Work out the finished part from the listing and answer in its coordinate system (mm). A direction names the side the tool comes from. Round coordinates to 2 decimals unless told otherwise and drop trailing zeros. Write each loop counter-clockwise with the first axis right and the second up, starting at its lowest first coordinate (ties: lowest second). Pieces come first, ordered by that corner, then holes. Notation, with made-up numbers: (-40, 51) -> (6, 51) arc R18 cw to (6, 78) -> close; hole circle Ø1 at (40, 87). An arc over 180 degrees is marked (long way). One line per question, with ' | ' between items. Start each with the question number.
```python
from build123d import *

# Parameters (mm, degrees)
SKETCH_1_W          = 64.2
SKETCH_1_H          = 33.2
EXTRUDE_1_DEPTH     = 2
SKETCH_2_W          = 61
SKETCH_2_H          = 29.5
SKETCH_2_W_2        = 59.4
SKETCH_2_H_2        = 27.9
EXTRUDE_2_DEPTH     = 5
OTHER_START         = -13.95
OTHER_1_OUTLINE_W   = 50.8
OTHER_1_OUTLINE_H   = 2
OTHER_1_DEPTH       = 19.2
OTHER_START_2       = 6.75
OTHER_1_2_OUTLINE_W = 20.2
OTHER_1_2_OUTLINE_H = 2
OTHER_1_2_DEPTH     = 7.2
EXTRUDE_6_DEPTH     = 5


# Read off the part's stored shape, not the designer's step: Полость1
with BuildPart() as part:
    # Эскиз1 → Бобышка-Вытянуть1 (new body)
    with BuildSketch(Plane(origin=(0, 0, 0), x_dir=(1, 0, 0), z_dir=(0, 1, 0))):
        Rectangle(SKETCH_1_W, SKETCH_1_H)
    extrude(amount=EXTRUDE_1_DEPTH)

    # Эскиз2 → Бобышка-Вытянуть2 (add)
    with BuildSketch(Plane(origin=(0, 2, 0), x_dir=(1, 0, 0), z_dir=(0, 1, 0))):
        Rectangle(SKETCH_2_W, SKETCH_2_H)
        Rectangle(SKETCH_2_W_2, SKETCH_2_H_2, mode=Mode.SUBTRACT)
    extrude(amount=EXTRUDE_2_DEPTH)

    # Полость1 outline → Полость1 (cut)
    with BuildSketch(Plane.XY.offset(OTHER_START)):
        with Locations((0, 1)):
            Rectangle(OTHER_1_OUTLINE_W, OTHER_1_OUTLINE_H)
    extrude(amount=OTHER_1_DEPTH, mode=Mode.SUBTRACT)

    # Other 1 2 outline → Other 1 2 (cut)
    with BuildSketch(Plane.XY.offset(OTHER_START_2)):
        with Locations((0, 1)):
            Rectangle(OTHER_1_2_OUTLINE_W, OTHER_1_2_OUTLINE_H)
    extrude(amount=OTHER_1_2_DEPTH, mode=Mode.SUBTRACT)

    # Эскиз8 → Бобышка-Вытянуть6 (add)
    with BuildSketch(Plane(origin=(0, 2, 0), x_dir=(1, 0, 0), z_dir=(0, 1, 0))):
        Polygon((-26.2, 13.95), (-26.2, -6.05), (-10.9, -6.05), (-10.9, -13.95), (-10.1, -13.95), (-10.1, -6.75), (10.1, -6.75), (10.1, -13.95), (10.9, -13.95), (10.9, -6.05), (26.2, -6.05), (26.2, 13.95), (25.4, 13.95), (25.4, -5.25), (-25.4, -5.25), (-25.4, 13.95), align=None)
    extrude(amount=EXTRUDE_6_DEPTH)


solid = part.part
```
(1) A cutting plane is placed at A-A, the plane z = 12. Determine the outline of the cut face in (x, y).
(2) The mould has two halves that part along Z. Classify faces 1 (the flat face through (28, 5, -13.95)), 2 (the flat face through (0, 4, 14.75)), 3 (the flat face through (-0.1, 7, 5.4)): +Z half, -Z half, draft (parallel to the pull), parting line (faces both ways), or undercut.
(3) A cutting plane is placed at B-B, the plane x = 22.5. Determine the outline of the cut face in (y, z), then the cut area to 3 significant figures.
(4) Given pin 1 Ø2.5 at (y, z) = (3.5, -3.5) entering from +X; pin 2 Ø1 at (x, y) = (-27.5, 5) entering from +Z; pin 3 Ø2.5 at (y, z) = (3.5, 9.5) entering from -X; pin 4 Ø10 at (x, z) = (-3.5, -3) entering from -Y, each flat-ended and moving along its own axis, determine where each tip first touches the part or whether it passes through.
(5) A cutting plane is placed at D-D, the plane x = 5.5. Determine the outline of the cut face in (y, z).
(6) A cutting plane is placed at C-C, the plane y = 0.75. Determine the outline of the cut face in (x, z).
(7) For faces 4 (the flat face through (-10.1, 3, 10)), 5 (the flat face through (0, 1, 16.6)), 6 (the flat face through (20, 5, 13.95)), 7 (the flat face through (0, 4, -14.75)), determine the directions among +Z, -Z, +X, -X, +Y, -Y from which every point of the face is accessible in a straight line to the end or side of a thin tool.
(8) Consider L1, parallel to X at y = 5, z = -1; L2, parallel to X at y = 2.5, z = 12; L3, parallel to Z at x = -20, y = 4.5. Determine where each line is inside the solid, lowest interval first.
Returned:
1) outline: (-32.1, 0) -> (-10.1, 0) -> (-10.1, 7) -> (-10.9, 7) -> (-10.9, 2) -> (-29.7, 2) -> (-29.7, 7) -> (-30.5, 7) -> (-30.5, 2) -> (-32.1, 2) -> close; (10.1, 0) -> (32.1, 0) -> (32.1, 2) -> (30.5, 2) -> (30.5, 7) -> (29.7, 7) -> (29.7, 2) -> (10.9, 2) -> (10.9, 7) -> (10.1, 7) -> close
2) face 1: undercut | face 2: +Z half | face 3: draft
3) outline: (0, -16.6) -> (2, -16.6) -> (2, -14.75) -> (7, -14.75) -> (7, -13.95) -> (0, -13.95) -> close; (0, 5.25) -> (7, 5.25) -> (7, 6.05) -> (2, 6.05) -> (2, 13.95) -> (7, 13.95) -> (7, 14.75) -> (2, 14.75) -> (2, 16.6) -> (0, 16.6) -> close | area: 40.0 mm2
4) pin 1: x = 30.5 | pin 2: z = 14.75 | pin 3: x = -30.5 | pin 4: through
5) outline: (0, -16.6) -> (2, -16.6) -> (2, -14.75) -> (7, -14.75) -> (7, -13.95) -> (0, -13.95) -> close; (0, 5.25) -> (7, 5.25) -> (7, 6.75) -> (0, 6.75) -> close; (0, 13.95) -> (7, 13.95) -> (7, 14.75) -> (2, 14.75) -> (2, 16.6) -> (0, 16.6) -> close
6) outline: (-32.1, -16.6) -> (32.1, -16.6) -> (32.1, 16.6) -> (-32.1, 16.6) -> close; hole (-25.4, -13.95) -> (25.4, -13.95) -> (25.4, 5.25) -> (-25.4, 5.25) -> close; hole (-10.1, 6.75) -> (10.1, 6.75) -> (10.1, 13.95) -> (-10.1, 13.95) -> close
7) face 4: +Y, -Y | face 5: +Z, +X, -X, +Y, -Y | face 6: +Y | face 7: -Z, +X, -X, +Y
8) L1: -30.5 to -29.7, -26.2 to -25.4, 25.4 to 26.2, 29.7 to 30.5 | L2: -30.5 to -29.7, -10.9 to -10.1, 10.1 to 10.9, 29.7 to 30.5 | L3: -14.75 to -13.95, 5.25 to 6.05, 13.95 to 14.75
